The listing builds one solid part. Answer for the finished solid, in the listing's coordinates (mm). Give positions to 0.01 mm unless a question says otherwise; leave off trailing zeros. Order: outer loops, then holes, each group sorted by start corner. A loop starts at its lowest first (then second) coordinate and runs counter-clockwise, first axis right, second up. Notation, with made-up numbers: (47, 83) - (87, 83) arc R21 cw to (87, 91) - close; hole circle Ø11 at (73, -16.75). An arc over 180 degrees is marked (long way). Answer as a JSON object with one key per item and string values. Group by question number.
Q1. Given pin 1 (12 mm diameter, centred on y = -20, z = 93, fed in from -X); pin 2 (1.5 mm diameter, centred on x = 2, z = 3, fed in from +Y); pin 3 (2 mm diameter, centred on x = 1.5, y = -22, fed in from +Z), each flat-ended and moving along its own axis, determine where each tip first touches the part or whether it passes through.
Q2. Consider line 1 (Y direction, x = 2.2, z = 17.5); line 2 (Z direction, x = 2.1, y = -25); line 3 (Y direction, x = 1.5, z = 48). Determine where each line is inside the solid, lowest interval first.
Q3. A cutting plane is placed at B-B, the plane z = -83. Give the vertices of the cut face in (x, y), and give its area (3 significant figures).
Q4. A cutting plane is placed at A-A, the plane x = 1.75. Count the separate pieces of the cut face and the enclosed holes in it, and give its area (3 significant figures).
Q5. A cutting plane is placed at C-C, the plane y = 6.5. Give the vertices of the cut face in (x, z).
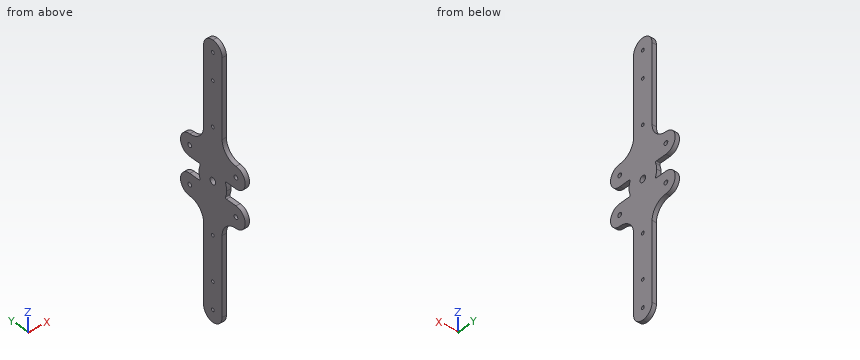
from build123d import *

# Parameters (mm, degrees)
SKETCH1_W            = 250
SKETCH1_H            = 75
BOSS_EXTRUDE1_DEPTH  = 4
SKETCH2_R            = 3
SKETCH2_R_2          = 1.5
CUT_EXTRUDE1_DEPTH   = 131.565117853
SKETCH3_R            = 2
CUT_EXTRUDE2_DEPTH   = 131.565117853
CUT_EXTRUDE3_DEPTH   = 131.565117853
FILLET1_R            = 1
FILLET1_OF_MIRROR2_R = 1
MIRROR3_OUTLINE_R    = 1.5
MIRROR3_OUTLINE_R_2  = 2
MIRROR3_DEPTH        = 4


# Read off the part's stored shape, not the designer's step: Mirror3
with BuildPart() as part:
    # Sketch1 → Boss-Extrude1 (new body)
    with BuildSketch(Plane(origin=(0, 0, 0), x_dir=(0, 0, -1), z_dir=(1, 0, 0))):
        Rectangle(SKETCH1_W, SKETCH1_H)
    extrude(amount=BOSS_EXTRUDE1_DEPTH)

    # Sketch2 → Cut-Extrude1 (cut, through all)
    with BuildSketch(Plane(origin=(4, 0, 0), x_dir=(0, 0, -1), z_dir=(1, 0, 0))):
        Circle(SKETCH2_R)
        with Locations((-48, 0)):
            Circle(SKETCH2_R_2)
        with Locations((-89, 0)):
            Circle(SKETCH2_R_2)
        with Locations((-114, 0)):
            Circle(SKETCH2_R_2)
    extrude(amount=-CUT_EXTRUDE1_DEPTH, mode=Mode.SUBTRACT)

    # Sketch3 → Cut-Extrude2 (cut, through all)
    with BuildSketch(Plane(origin=(4, 0, 0), x_dir=(0, 0, -1), z_dir=(1, 0, 0))):
        with Locations((-17.5, 25)):
            Circle(SKETCH3_R)
    cut_extrude2 = extrude(amount=-CUT_EXTRUDE2_DEPTH, mode=Mode.SUBTRACT)

    # Sketch4 → Cut-Extrude3 (cut, through all)
    with BuildSketch(Plane(origin=(4, 0, 0), x_dir=(0, 0, -1), z_dir=(1, 0, 0))):
        with BuildLine():
            Line((-115, 10), (-42.5, 10))
            ThreePointArc((-42.5, 10), (-31.893398282, 14.393398282), (-27.5, 25))
            ThreePointArc((-27.5, 25), (-17.5, 35), (-7.5, 25))
            Line((-7.5, 25), (-7.5, 13))
            ThreePointArc((-7.5, 13), (-3.882119057, 14.497556747), (0, 15.00833102))
            Line((0, 15.00833102), (0, 37.5))
            Line((0, 37.5), (-125, 37.5))
            Line((-125, 37.5), (-125, 0))
            ThreePointArc((-125, 0), (-122.071067812, 7.071067812), (-115, 10))
        make_face()
    cut_extrude3 = extrude(amount=-CUT_EXTRUDE3_DEPTH, mode=Mode.SUBTRACT)

    # Fillet1
    fillet1_edges = [part.edges().sort_by_distance(p)[0] for p in [
        (2, 13, 7.5),
    ]]
    fillet(fillet1_edges, radius=FILLET1_R)

    # Mirror2: Cut-Extrude2, Cut-Extrude3 across plane
    add(cut_extrude2.mirror(Plane.ZX), mode=Mode.SUBTRACT)
    add(cut_extrude3.mirror(Plane.ZX), mode=Mode.SUBTRACT)

    # Fillet1 of Mirror2
    fillet1_of_mirror2_edges = [part.edges().sort_by_distance(p)[0] for p in [
        (2, -13, 7.5),
    ]]
    fillet(fillet1_of_mirror2_edges, radius=FILLET1_OF_MIRROR2_R)

    # Mirror3 outline → Mirror3 (cut)
    with BuildSketch(Plane.YZ):
        with BuildLine():
            Line((-37.5, -125), (-3.5e-08, -125))
            ThreePointArc((-3.5e-08, -125), (-7.071067824, -122.071067799), (-10, -115))
            Line((-10, -115), (-10, -42.5))
            ThreePointArc((-10, -42.5), (-14.393398282, -31.893398282), (-25, -27.5))
            ThreePointArc((-25, -27.5), (-35, -17.5), (-25, -7.5))
            Line((-25, -7.5), (-14.629308324, -7.5))
            ThreePointArc((-14.629308324, -7.5), (-13.790845868, -7.044959365), (-13.715452388, -6.09396142))
            ThreePointArc((-13.715452388, -6.09396142), (-14.681553895, -3.114799389), (-15.00833102, 0))
            Line((-15.00833102, 0), (-37.5, 0))
            Line((-37.5, 0), (-37.5, -125))
        make_face()
        with BuildLine():
            ThreePointArc((15.00833102, 0), (14.681553895, -3.114799389), (13.715452388, -6.09396142))
            ThreePointArc((13.715452388, -6.09396142), (13.790845868, -7.044959365), (14.629308324, -7.5))
            Line((14.629308324, -7.5), (25, -7.5))
            ThreePointArc((25, -7.5), (35, -17.5), (25, -27.5))
            ThreePointArc((25, -27.5), (14.393398282, -31.893398282), (10, -42.5))
            Line((10, -42.5), (10, -115))
            ThreePointArc((10, -115), (7.071067799, -122.071067824), (-3.5e-08, -125))
            Line((-3.5e-08, -125), (37.5, -125))
            Line((37.5, -125), (37.5, 0))
            Line((37.5, 0), (15.00833102, 0))
        make_face()
        with Locations((0, -114)):
            Circle(MIRROR3_OUTLINE_R)
        with Locations((0, -89)):
            Circle(MIRROR3_OUTLINE_R)
        with Locations((0, -48)):
            Circle(MIRROR3_OUTLINE_R)
        with Locations((25, -17.5)):
            Circle(MIRROR3_OUTLINE_R_2)
        with Locations((-25, -17.5)):
            Circle(MIRROR3_OUTLINE_R_2)
    extrude(amount=MIRROR3_DEPTH, mode=Mode.SUBTRACT)


solid = part.part
Reply:
{
 "1": {"pin 1": "passes through", "pin 2": "stops at y = 14.84", "pin 3": "stops at z = 28.04"},
 "2": {"line 1": "y = -35 to -27, -23 to 23, 27 to 35", "line 2": "z = -27.5 to -19.5, -15.5 to -7.5, 7.5 to 15.5, 19.5 to 27.5", "line 3": "y = -10 to -1.5, 1.5 to 10"},
 "3": {"outline": "(0, -10) - (4, -10) - (4, 10) - (0, 10) - close", "area": "80.0 mm^2"},
 "4": {"separate pieces": "1", "enclosed holes": "11", "area": "6,950 mm^2"},
 "5": {"outline": "(0, -122.6) - (4, -122.6) - (4, 122.6) - (0, 122.6) - close"}
}
